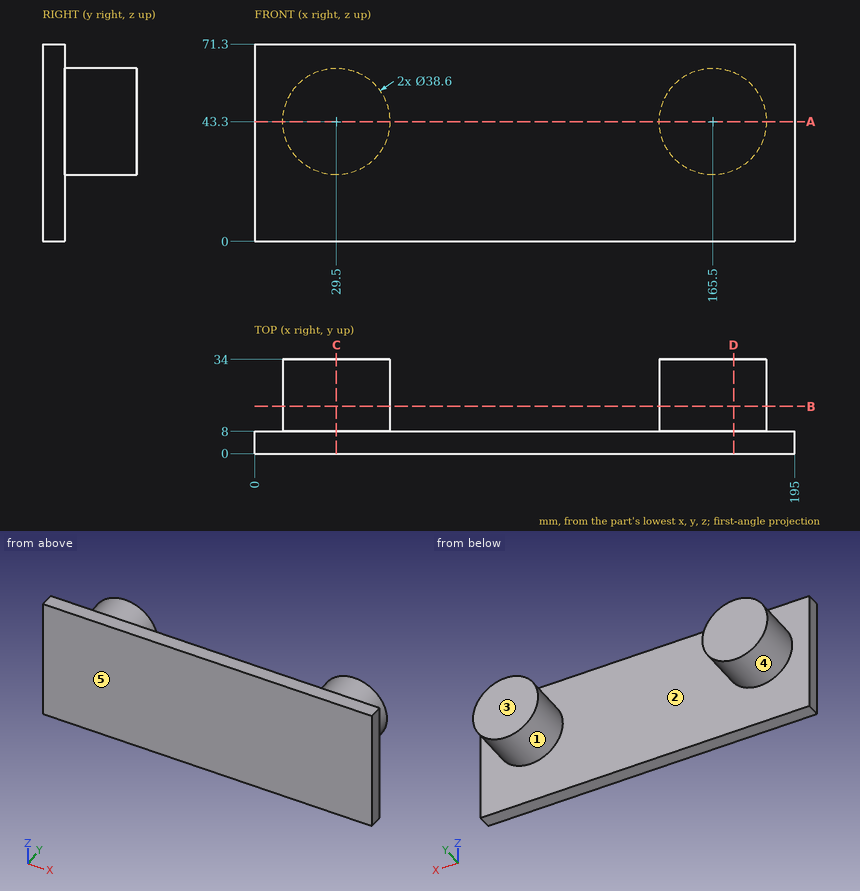
For this review, use the dimensioned drawing (mm, ordinates from the lowest corner) and the shaded views. A direction names the side the tool comes from. Round coordinates to 2 decimals unless told otherwise and drop trailing zeros. Order: outer loops, then holes, each group sorted by start corner. A loop starts at its lowest first (then second) coordinate and runs counter-clockwise, first axis right, second up. Notation, with made-up numbers: (-28.75, 73) -> (-16.75, 73) arc R27 ccw to (-16.75, 106) -> close; hole circle Ø5 at (64, 84). An arc over 180 degrees is marked (long way). One line per item, written item: value. Start each with the question number.
Q1. Take a section at B-B (y = 17). Write out the cut boundary in (x, z), and give its area (3 significant figures).
Q2. Machinability: for the marked faces 4 and 5, which of the approach directions +Z, -Z, +X, -X, +Y, -Y give a long, thin tool a straight path to every point of the face, cutting with its end or side? Answer none if there is none.
Q3. Take a section at D-D (x = 173). Write out the cut boundary in (y, z).
Q4. Mouldability with a two-part tool opening along X and no side actions: class the marked faces 1, 2 and 3 as released by +X, released by -X, zero draft, split by the parting line, or undercut.
Q5. Clearance check with flat-ended pins moving along their axes: pin 1 Ø1.5 at (x, z) = (113.5, 42) entering from -Y; pin 2 Ø6 at (y, z) = (12, 30.5) entering from +X; pin 3 Ø1.5 at (y, z) = (11, 33) entering from +X; pin 4 Ø6 at (x, z) = (64, 47.5) entering from +Y. State where each tip first meets the part, or that it passes through.
Q6. Take a section at C-C (x = 29.5). Write out the cut boundary in (y, z), and give its area (3 significant figures).
Q7. Take a section at A-A (z = 43.3). Write out the cut boundary in (x, y), and give its area (3 significant figures).
Q8. Wall thickness on line 1 (Y direction, x = 142, z = 67); line 2 (X direction, y = 15, z = 28); line 3 (Z direction, x = 166, y = 28.5): over which ranges is each line inside the solid? List them lowest first.
Reported:
1. outline: circle Ø38.6 at (29.5, 43.3); circle Ø38.6 at (165.5, 43.3)
1. area: 2,340 mm2
2. face 4: +Y
2. face 5: +Z, -Z, +X, -X, -Y
3. outline: (0, 0) -> (8, 0) -> (8, 25.52) -> (34, 25.52) -> (34, 61.08) -> (8, 61.08) -> (8, 71.3) -> (0, 71.3) -> close
4. face 1: undercut
4. face 2: undercut
4. face 3: zero draft
5. pin 1: stops at y = 0
5. pin 2: stops at x = 182.13
5. pin 3: stops at x = 182.27
5. pin 4: stops at y = 8
6. outline: (0, 0) -> (8, 0) -> (8, 24) -> (34, 24) -> (34, 62.6) -> (8, 62.6) -> (8, 71.3) -> (0, 71.3) -> close
6. area: 1,570 mm2
7. outline: (0, 0) -> (195, 0) -> (195, 8) -> (184.8, 8) -> (184.8, 34) -> (146.2, 34) -> (146.2, 8) -> (48.8, 8) -> (48.8, 34) -> (10.2, 34) -> (10.2, 8) -> (0, 8) -> close
7. area: 3,570 mm2
8. line 1: y = 0 to 8
8. line 2: x = 17.74 to 41.26, 153.74 to 177.26
8. line 3: z = 24.01 to 62.59
